```python
from build123d import *

# Parameters (mm, degrees)
SKETCH_1_R          = 3
EXTRUDE_1_DEPTH     = 15
SKETCH_2_R          = 4
CUT_EXTRUDE_1_DEPTH = 3
SKETCH_3_R          = 2.5
CUT_EXTRUDE_2_DEPTH = 15
SKETCH_4_R          = 5
CUT_EXTRUDE_3_DEPTH = 6


with BuildPart() as part:
    # 草图1 → 凸台-拉伸1 (new body)
    with BuildSketch(Plane.XY):
        with BuildLine():
            Line((-50, 0), (0, 0))
            Line((0, 0), (0, -20))
            Line((0, -20), (-50, -20))
            ThreePointArc((-50, -20), (-60, -10), (-50, 0))
        make_face()
        with Locations((-25, -10)):
            Circle(SKETCH_1_R, mode=Mode.SUBTRACT)
        with Locations((-10, -10)):
            Circle(SKETCH_1_R, mode=Mode.SUBTRACT)
    extrude(amount=EXTRUDE_1_DEPTH)

    # 草图2 → 切除-拉伸1 (cut)
    with BuildSketch(Plane.XY.offset(15)):
        with Locations((-50, -10)):
            Circle(SKETCH_2_R)
    extrude(amount=-CUT_EXTRUDE_1_DEPTH, mode=Mode.SUBTRACT)

    # 草图3 → 切除-拉伸2 (cut)
    with BuildSketch(Plane.XY.offset(12)):
        with Locations((-50, -10)):
            Circle(SKETCH_3_R)
    extrude(amount=-CUT_EXTRUDE_2_DEPTH, mode=Mode.SUBTRACT)

    # 草图4 → 切除-拉伸3 (cut)
    with BuildSketch(Plane(origin=(0, 0, 0), x_dir=(-1, 0, 0), z_dir=(0, 0, -1))):
        with Locations((10, -10)):
            Circle(SKETCH_4_R)
        with Locations((25, -10)):
            Circle(SKETCH_4_R)
    extrude(amount=-CUT_EXTRUDE_3_DEPTH, mode=Mode.SUBTRACT)


solid = part.part
```
Source: CAD feature listing. Evaluate the final solid. Frame: model axes, mm. A direction names the side the tool comes from. Round coordinates to 2 decimals unless told otherwise and drop trailing zeros. Loops run counter-clockwise (first coordinate to the right, second up) from the corner with the lowest first, then second, coordinate; pieces in that order, holes last.
(1) Section query D-D (z = 5.25). Output: boundary loops of the cut face in (x, y), and give its area (3 significant figures).
From the geometry:
outline: (-50, -20) - (0, -20) - (0, 0) - (-50, 0) arc R10 ccw to start; hole circle Ø5 at (-50, -10); hole circle Ø10 at (-25, -10); hole circle Ø10 at (-10, -10)
area: 980 mm2
(2) Material intervals for probe 1 along X at (y, z) = (-10.25, 9.25); probe 2 along X at (y, z) = (-7.75, 9.25); probe 3 along Y at (x, z) = (-50, 13.5), sorted ascending.
From the geometry:
probe 1: x = -60 to -52.49, -47.51 to -27.99, -22.01 to -12.99, -7.01 to 0
probe 2: x = -59.74 to -51.09, -48.91 to -26.98, -23.02 to -11.98, -8.02 to 0
probe 3: y = -20 to -14, -6 to 0
(3) Section query B-B (x = -25). Output: boundary loops of the cut face in (y, z), and give its area (3 significant figures).
From the geometry:
outline: (-20, 0) - (-15, 0) - (-15, 6) - (-13, 6) - (-13, 15) - (-20, 15) - close; (-7, 6) - (-5, 6) - (-5, 0) - (0, 0) - (0, 15) - (-7, 15) - close
area: 186 mm2
(4) Pull-direction query (X, two-part tool) for faces 1 (the flat face through (-30, -8, 0)), 2 (the cylindrical face through (-12.21, -7.97, 10.44)), 3 (the cylindrical face through (-60, -10, 7)); classes: +X half, -X half, draft (parallel to the pull), parting line (faces both ways), or undercut.
From the geometry:
face 1: draft
face 2: undercut
face 3: -X half
(5) Section query C-C (z = 13.75). Output: boundary loops of the cut face in (x, y).
From the geometry:
outline: (-50, -20) - (0, -20) - (0, 0) - (-50, 0) arc R10 ccw to start; hole circle Ø8 at (-50, -10); hole circle Ø6 at (-25, -10); hole circle Ø6 at (-10, -10)
(6) Access query for faces 4 (the flat face through (-30, -10, 15)), 5 (the flat face through (-24.9, -13.3, 6)), 6 (the flat face through (-48, -8, 12)). Directions: +Z, -Z, +X, -X, +Y, -Y. A direction counts if a zero-diameter tool reaches every point of the face in a straight line with its end or side. Return the directions, or none.
From the geometry:
face 4: +Z, +X, -X, +Y, -Y
face 5: -Z
face 6: +Z
(7) Section query A-A (y = -10). Output: boundary loops of the cut face in (x, z), and give its area (3 significant figures).
From the geometry:
outline: (-60, 0) - (-52.5, 0) - (-52.5, 12) - (-54, 12) - (-54, 15) - (-60, 15) - close; (-47.5, 0) - (-30, 0) - (-30, 6) - (-28, 6) - (-28, 15) - (-46, 15) - (-46, 12) - (-47.5, 12) - close; (-22, 6) - (-20, 6) - (-20, 0) - (-15, 0) - (-15, 6) - (-13, 6) - (-13, 15) - (-22, 15) - close; (-7, 6) - (-5, 6) - (-5, 0) - (0, 0) - (0, 15) - (-7, 15) - close
area: 588 mm2
(8) Contact query for flat-ended pins moving along their axis: pin 1 Ø7 at (x, y) = (-10, -10) entering from -Z; pin 2 Ø4 at (x, y) = (-50, -11) entering from +Z; pin 3 Ø6 at (y, z) = (-13.5, 2.5) entering from -X; pin 4 Ø4 at (x, y) = (-50, -10) entering from +Z. Output: stop coordinate, or through.
From the geometry:
pin 1: stops at z = 6
pin 2: stops at z = 12
pin 3: stops at x = -59.99
pin 4: passes through
